Part model, mm, in its own coordinate system. Face numbers are marked on the shaded views. Round coordinates to 2 decimals unless told otherwise and drop trailing zeros. Write each loop counter-clockwise with the first axis right and the second up, starting at its lowest first coordinate (ties: lowest second). Pieces come first, ordered by that corner, then holes.
```python
from build123d import *

# Parameters (mm, degrees)
BOSS_EXTRUDE1_DEPTH           = 9.5
BOSS_EXTRUDE1_DEPTH_BACK      = 9.5
SKETCH1_R                     = 90
CSK_FOR_M8_SFHCS2_D           = 17.5
CSK_FOR_M8_SFHCS2_CSINK_D     = 17.92
CSK_FOR_M8_SFHCS2_CSINK_ANGLE = 90
SKETCH8_R                     = 4
CUT_EXTRUDE3_DEPTH            = 128.633263689
CIRPATTERN2_COUNT             = 4


with BuildPart() as part:
    # Sketch1 → Boss-Extrude1 (new, two sides: drawn at the far end of the back side and taken through both)
    with BuildSketch(Plane(origin=(0, 0, 0), x_dir=(1, 0, 0), z_dir=(0, 1, 0)).offset(-BOSS_EXTRUDE1_DEPTH_BACK)):
        with Locations(Location((0, 0, 0), (0, 0, 270))):
            Circle(SKETCH1_R)
    extrude(amount=BOSS_EXTRUDE1_DEPTH + BOSS_EXTRUDE1_DEPTH_BACK)

    # CSK for M8 SFHCS2 (through all)
    with Locations(Plane(origin=(0, -9.5, 0), x_dir=(-1, 0, 0), z_dir=(0, -1, 0))):
        with Locations((0, 0)):
            CounterSinkHole(CSK_FOR_M8_SFHCS2_D / 2, CSK_FOR_M8_SFHCS2_CSINK_D / 2, counter_sink_angle=CSK_FOR_M8_SFHCS2_CSINK_ANGLE)

    # Sketch8 → Cut-Extrude3 (cut, symmetric)
    with BuildSketch(Plane(origin=(0, 0, 0), x_dir=(1, 0, 0), z_dir=(0, 1, 0))):
        with Locations(Location((26.787840266, 64.671567276, 0), (0, 0, 270))):
            Circle(SKETCH8_R)
    cut_extrude3 = extrude(amount=CUT_EXTRUDE3_DEPTH, both=True, mode=Mode.SUBTRACT)

    # CirPattern2: Cut-Extrude3 ×4 about axis
    cirpattern2_axis = Axis((0, 0, 0), (0, 1, 0))
    for i in range(1, CIRPATTERN2_COUNT):
        add(cut_extrude3.rotate(cirpattern2_axis, i * 360 / CIRPATTERN2_COUNT), mode=Mode.SUBTRACT)


solid = part.part
```
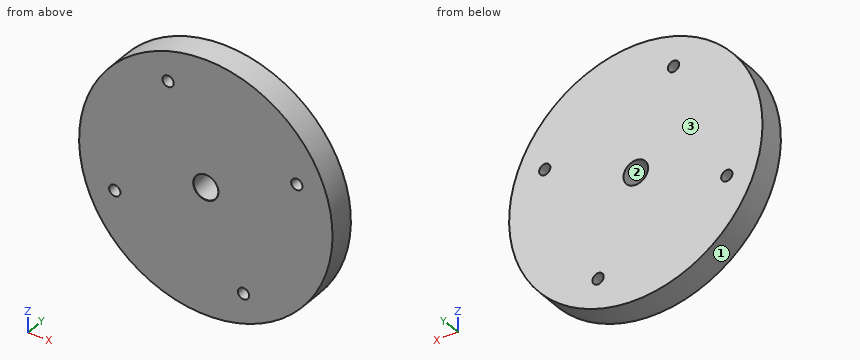
Q1. Drop flat-ended pins along their axis: pin 1 (8 mm diameter, centred on x = 61.5, y = 4.5, fed in from +Z); pin 2 (1.5 mm diameter, centred on x = 23.5, y = -7.5, fed in from +Z); pin 3 (3 mm diameter, centred on x = -44.5, y = -4.5, fed in from -Z). Give the stop position or say it passes through.
Values follow:
pin 1: stops at z = 69.24
pin 2: stops at z = 87.08
pin 3: stops at z = -79.06
Q2. Cut at A-A on x = 0. Write the cut outline in (y, z), plus the area to 3 significant figures.
Values follow:
outline: (-9.5, -90) - (9.5, -90) - (9.5, -8.75) - (-9.29, -8.75) - (-9.5, -8.96) - close; (-9.5, 8.96) - (-9.29, 8.75) - (9.5, 8.75) - (9.5, 90) - (-9.5, 90) - close
area: 3,090 mm2
Q3. Cut at B-B on z = -63.5. Write the cut outline in (x, y).
Values follow:
outline: (-63.78, -9.5) - (22.96, -9.5) - (22.96, 9.5) - (-63.78, 9.5) - close; (30.61, -9.5) - (63.78, -9.5) - (63.78, 9.5) - (30.61, 9.5) - close
Q4. Cut at D-D on y = -4.75. Write the cut outline in (x, z).
Values follow:
outline: circle Ø180 at (0, 0); hole circle Ø8 at (-64.67, -26.79); hole circle Ø8 at (-26.79, 64.67); hole circle Ø17.5 at (0, 0); hole circle Ø8 at (26.79, -64.67); hole circle Ø8 at (64.67, 26.79)
Q5. Cut at C-C on z = 0. Write the cut outline in (x, y), plus the area to 3 significant figures.
Values follow:
outline: (-90, -9.5) - (-8.96, -9.5) - (-8.75, -9.29) - (-8.75, 9.5) - (-90, 9.5) - close; (8.75, -9.29) - (8.96, -9.5) - (90, -9.5) - (90, 9.5) - (8.75, 9.5) - close
area: 3,090 mm2
Q6. Wall check: L1, parallel to X at y = -3.25, z = 25.5; L2, parallel to X at y = 1.5, z = -6; L3, parallel to Z at x = -63, y = -3.25. Give the ranges that are in metal, low to high.
Values follow:
L1: x = -86.31 to 60.88, 68.46 to 86.31
L2: x = -89.8 to -6.37, 6.37 to 89.8
L3: z = -64.27 to -30.42, -23.15 to 64.27
Q7. Mould opens along Z. For the marked faces 1, 2 and 3 say: +Z half, -Z half, draft (parallel to the pull), parting line (faces both ways), or undercut.
Values follow:
face 1: parting line
face 2: undercut
face 3: draft
